```python
from build123d import *

# Parameters (mm, degrees)
EXTRUDE_1_DEPTH     = 19
SKETCH_2_R          = 5
CUT_EXTRUDE_1_DEPTH = 2
SKETCH_3_R          = 1.5
CUT_EXTRUDE_2_DEPTH = 10


with BuildPart() as part:
    # 草圖1 → 填料-伸長1 (new body)
    with BuildSketch(Plane.XY):
        with BuildLine():
            Line((-16, 0), (-16, -25))
            Line((-16, -25), (16, -25))
            Line((16, -25), (16, 0))
            ThreePointArc((16, 0), (0, 16), (-16, 0))
        make_face()
    extrude(amount=EXTRUDE_1_DEPTH)

    # 草圖2 → 除料-伸長1 (cut)
    with BuildSketch(Plane(origin=(0, 0, 0), x_dir=(-1, 0, 0), z_dir=(0, 0, -1))):
        Circle(SKETCH_2_R)
    extrude(amount=-CUT_EXTRUDE_1_DEPTH, mode=Mode.SUBTRACT)

    # 草圖3 → 除料-伸長2 (cut)
    with BuildSketch(Plane(origin=(0, 0, 2), x_dir=(-1, 0, 0), z_dir=(0, 0, -1))):
        Circle(SKETCH_3_R)
    extrude(amount=-CUT_EXTRUDE_2_DEPTH, mode=Mode.SUBTRACT)


solid = part.part
```
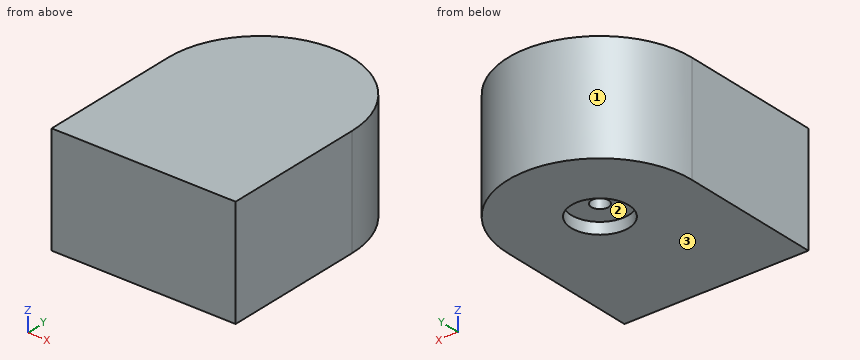
The model under review builds one solid part; all positions refer to its coordinate system, in mm. Face numbers are marked on the shaded views. Round coordinates to 2 decimals unless told otherwise and drop trailing zeros. Order: outer loops, then holes, each group sorted by start corner. A loop starts at its lowest first (then second) coordinate and runs counter-clockwise, first axis right, second up. Notation, with made-up numbers: M 59.5,32 L 68.5,32 A18 cw 68.5,54 Z; hole C 53.5,-25.75 d1. An arc over 180 degrees is marked long. Use a Markdown table: item, result.
1) Draft analysis for pull direction Y (two halves, no side actions). For the marked faces 1, 2 and 3, state which applies: released by +Y, released by -Y, zero draft, split by the parting line, or undercut.
Report:
| item | result |
|---|---|
| face 1 | released by +Y |
| face 2 | undercut |
| face 3 | zero draft |
2) Consider section C-C (x = 0). Write out the cut boundary in (y, z).
Report:
| item | result |
|---|---|
| outline | M -25,0 L -5,0 L -5,2 L -1.5,2 L -1.5,12 L 1.5,12 L 1.5,2 L 5,2 L 5,0 L 16,0 L 16,19 L -25,19 Z |
3) Wall thickness on line 1 along Y through (x, z) = (0, 0.95); line 2 along Y through (x, z) = (0, 4.75); line 3 along Y through (x, z) = (3, 11.25): over which ranges is each line inside the solid? List them lowest first. Write a range as [from, to].
Report:
| item | result |
|---|---|
| line 1 | [-25, -5], [5, 16] |
| line 2 | [-25, -1.5], [1.5, 16] |
| line 3 | [-25, 15.72] |
4) Consider section B-B (y = -3). Write out the cut boundary in (x, z).
Report:
| item | result |
|---|---|
| outline | M -16,0 L -4,0 L -4,2 L 4,2 L 4,0 L 16,0 L 16,19 L -16,19 Z |
5) Consider section D-D (y = 8.5). Write out the cut boundary in (x, z).
Report:
| item | result |
|---|---|
| outline | M -13.56,0 L 13.56,0 L 13.56,19 L -13.56,19 Z |
6) Consider section A-A (z = 4.75). Write out the cut boundary in (x, y).
Report:
| item | result |
|---|---|
| outline | M -16,-25 L 16,-25 L 16,0 A16 ccw -16,0 Z; hole C 0,0 d3 |
7) Insertion check: pin 1 (1.8 mm diameter, centred on x = 0, y = 0, fed in from -Z); pin 2 (1.5 mm diameter, centred on y = 5, z = 8.5, fed in from +X); pin 3 (8 mm diameter, centred on x = 0, y = -0.5, fed in from -Z). Each pin has a flat end and moves straight along its axis. Give the tip position at first contact, or say it passes through.
Report:
| item | result |
|---|---|
| pin 1 | z = 12 |
| pin 2 | x = 15.43 |
| pin 3 | z = 2 |
